Design review of the part shown in the three views and the two pictorial views. Dimensions are in mm from the part's minimum x, y and z. Round coordinates to 2 decimals unless told otherwise and drop trailing zeros. Order: outer loops, then holes, each group sorted by start corner. A loop starts at its lowest first (then second) coordinate and runs counter-clockwise, first axis right, second up. Notation, with made-up numbers: (85, 65) - (143, 65) arc R17 ccw to (143, 87) - close; hole circle Ø2 at (-29, 24.5). An arc over 180 degrees is marked (long way). One line per item, written item: value.
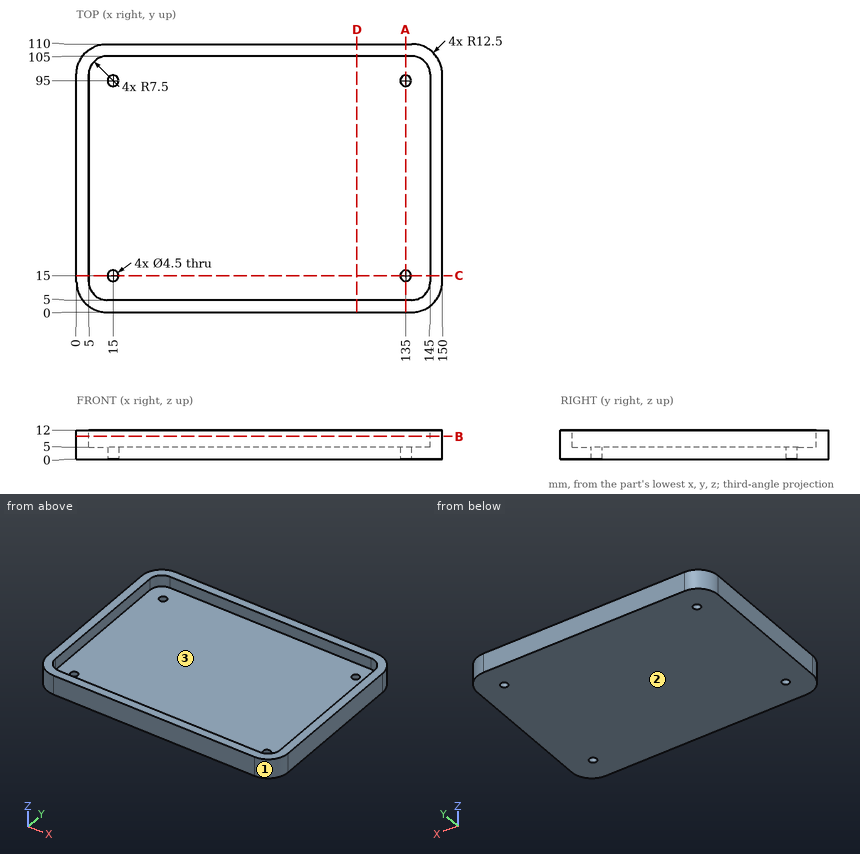
Item 1: For P1, Ø4, axis at x = 93, y = 71.5, coming from the +Z side, flat-tipped, find the tip position at first contact; note if it passes through.
Returned:
P1: z = 5
Item 2: Take a section at B-B (z = 9.5). Write out the cut boundary in (x, y).
Returned:
outline: (0, 12.5) arc R12.5 ccw to (12.5, 0) - (137.5, 0) arc R12.5 ccw to (150, 12.5) - (150, 97.5) arc R12.5 ccw to (137.5, 110) - (12.5, 110) arc R12.5 ccw to (0, 97.5) - close; hole (5, 12.5) arc R7.5 ccw to (12.5, 5) - (137.5, 5) arc R7.5 ccw to (145, 12.5) - (145, 97.5) arc R7.5 ccw to (137.5, 105) - (12.5, 105) arc R7.5 ccw to (5, 97.5) - close
Item 3: Take a section at D-D (x = 115). Write out the cut boundary in (y, z), plus the area to 3 significant figures.
Returned:
outline: (0, 0) - (110, 0) - (110, 12) - (105, 12) - (105, 5) - (5, 5) - (5, 12) - (0, 12) - close
area: 620 mm^2
Item 4: The part is to be moulded in two halves that separate along Z. For the marked faces 1, 2 and 3, say which applies: +Z half, -Z half, draft (parallel to the pull), parting line (faces both ways), or undercut.
Returned:
face 1: draft
face 2: -Z half
face 3: +Z half
Item 5: Take a section at A-A (x = 135). Write out the cut boundary in (y, z).
Returned:
outline: (0, 0) - (12.75, 0) - (12.75, 5) - (5, 5) - (5, 12) - (0, 12) - close; (17.25, 0) - (92.75, 0) - (92.75, 5) - (17.25, 5) - close; (97.25, 0) - (110, 0) - (110, 12) - (105, 12) - (105, 5) - (97.25, 5) - close
Item 6: Take a section at C-C (y = 15). Write out the cut boundary in (x, z), plus the area to 3 significant figures.
Returned:
outline: (0, 0) - (12.75, 0) - (12.75, 5) - (5, 5) - (5, 12) - (0, 12) - close; (17.25, 0) - (132.75, 0) - (132.75, 5) - (17.25, 5) - close; (137.25, 0) - (150, 0) - (150, 12) - (145, 12) - (145, 5) - (137.25, 5) - close
area: 775 mm^2
Item 7: Wall thickness on line 1 (X direction, y = 95, z = 1.5); line 2 (Y direction, x = 135, z = 2.4); line 3 (X direction, y = 37, z = 10): over which ranges is each line inside the solid? List them lowest first.
Returned:
line 1: 0 to 12.75, 17.25 to 132.75, 137.25 to 150
line 2: 0 to 12.75, 17.25 to 92.75, 97.25 to 110
line 3: 0 to 5, 145 to 150
